```python
from build123d import *

# Parameters (mm, degrees)
F0_R     = 12.7
F1_DEPTH = 609.6
F2_R     = 19.05
F2_R_2   = 12.7
F3_DEPTH = 127
F4_W     = 50.8
F4_H     = 50.8
F5_DEPTH = 12.7
F6_R     = 15.875
F7_DEPTH = 12.7


with BuildPart() as f1:
    # F0 (on Front) → F1 (new body)
    with BuildSketch(Plane.XZ):
        Circle(F0_R)
    extrude(amount=F1_DEPTH)

    # F2 (on face) → F3 (join)
    with BuildSketch(Plane.XZ.offset(609.6)):
        Circle(F2_R)
        Circle(F2_R_2, mode=Mode.SUBTRACT)
        Circle(F2_R_2)
    extrude(amount=F3_DEPTH)

    # F4 (on Right) → F5 (join, symmetric)
    with BuildSketch(Plane.YZ):
        with Locations((25.4, 0)):
            Rectangle(F4_W, F4_H)
    extrude(amount=F5_DEPTH, both=True)

    # F6 (on face) → F7 (join)
    with BuildSketch(Plane(origin=(-12.7, 0, 0), x_dir=(0, -1, 0), z_dir=(-1, 0, 0))):
        with Locations((-25.4, 0)):
            Circle(F6_R)
    extrude(amount=F7_DEPTH)


solid = f1.part
```
Geometry: final body of the model. Coordinates: model frame, mm. A direction names the side the tool comes from. Give positions to 0.01 mm unless a question says otherwise; leave off trailing zeros. Loops run counter-clockwise (first coordinate to the right, second up) from the corner with the lowest first, then second, coordinate; pieces in that order, holes last. Notation, with made-up numbers: (77, 28) -> (92, 28) arc R15 cw to (92, 35) -> close; hole circle Ø9 at (-38.5, -1). An arc over 180 degrees is marked (long way). Use CSV: the item, a comma, the result in double quotes.
(1) Cut plane B-B (x = 0). Output: boundary loops of the cut face in (y, z).
From the geometry:
outline,"(-736.6, -19.05) -> (-609.6, -19.05) -> (-609.6, -12.7) -> (0, -12.7) -> (0, -25.4) -> (50.8, -25.4) -> (50.8, 25.4) -> (0, 25.4) -> (0, 12.7) -> (-609.6, 12.7) -> (-609.6, 19.05) -> (-736.6, 19.05) -> close"
(2) Access query for faces 1 (the face through (12.7, 25, 0)), 2 (the face through (0, 0, 18)), 3 (the face through (-18.96, 41.26, 0.7)). Directions: +Z, -Z, +X, -X, +Y, -Y. A direction counts if a zero-diameter tool reaches every point of the face in a straight line with its end or side. Return the directions, or none.
From the geometry:
face 1,"+Z, -Z, +X, +Y"
face 2,"+Z"
face 3,"-X"
(3) Pull-direction query (Y, two-part tool) for faces 4 (the face through (0, -736.6, 0)), 5 (the face through (-15.12, -672.21, -11.59)), 6 (the face through (4, -609.6, -12.4)); classes: released by +Y, released by -Y, zero draft, split by the parting line, or undercut.
From the geometry:
face 4,"released by -Y"
face 5,"zero draft"
face 6,"undercut"
(4) First-contact query: P1, Ø1.5, axis at y = -449, z = -11.5, coming from the -X side; P2, Ø15, axis at y = 36, z = 8.5, coming from the +X side; P3, Ø4, axis at x = -5.5, y = -657, coming from the +Z side; P4, Ø10, axis at x = -16.5, z = -10.5, coming from the +Y side. Flat tips, straight axial feed; report the tip coordinate or a pass-through.
From the geometry:
P1,"x = -6.76"
P2,"x = 12.7"
P3,"z = 18.73"
P4,"y = 50.8"
(5) Cut plane C-C (y = -72). Output: boundary loops of the cut face in (x, z).
From the geometry:
outline,"circle Ø25.4 at (0, 0)"
(6) Cut plane A-A (y = 25.4). Output: boundary loops of the cut face in (x, z) (3 decimals).
From the geometry:
outline,"(-25.4, -15.875) -> (-12.7, -15.875) -> (-12.7, -25.4) -> (12.7, -25.4) -> (12.7, 25.4) -> (-12.7, 25.4) -> (-12.7, 15.875) -> (-25.4, 15.875) -> close"
(7) Ray query, line 1 along Z through (x, y) = (0.5, -169); line 2 along Y through (x, z) = (-10, 15); line 3 along Y through (x, z) = (-4, 19). Return the intervals inside material, ascending. Write a range as [from, to].
From the geometry:
line 1,"[-12.69, 12.69]"
line 2,"[-736.6, -609.6], [0, 50.8]"
line 3,"[0, 50.8]"
